Can you work these out from the model? Positions are in its coordinate system, mm. A direction names the side the tool comes from. Round coordinates to 2 decimals unless told otherwise and drop trailing zeros. Write each loop counter-clockwise with the first axis right and the second up, starting at its lowest first coordinate (ties: lowest second). Pieces come first, ordered by that corner, then holes. Notation, with made-up numbers: M 55.5,36.25 L 99.5,36.25 A20 cw 99.5,62.25 Z; hole C 48,45.5 d10. An arc over 180 degrees is marked long. Answer in a Markdown table with one row per item. Add a question column.
(1) Suppose I cut it at C-C, the plane z = -1.75. Write out the boundary of the cut face in (x, y).
(2) If I drill on probe 1 along X at (y, z) = (6.5, 8.5); probe 2 along X at (y, z) = (-1, -5.5); probe 3 along Z at (x, y) = (-15, 4.5), over which ranges is the centre line in solid material (lowest first)?
(3) Suppose I cut it at B-B, the plane y = 15. Write out the boundary of the cut face in (x, z), then the cut area to 3 significant figures.
(4) If we mould it in two halves opening along Y, with no side actions, what happens to faces 4 (the face through (0, -20, 0)), 5 (the face through (20.25, 0, 0)), 6 (the face through (-13, 10, -9))? For each: released by +Y, released by -Y, zero draft, split by the parting line, or undercut.
(5) For faces 1 (the face through (23.97, 12.54, -1.05)), 2 (the face through (-13, 0, 9)), 3 (the face through (-21.75, 7, 0)), which set-ups out of +Z, -Z, +X, -X, +Y, -Y let a thin tool reach every point of the face, with its end or its side?
(6) I'm going to push flat-ended pins straight in: pin 1 (0.6 mm diameter, centred on y = 4, z = -9, fed in from +X); pin 2 (4 mm diameter, centred on y = 6.5, z = 3, fed in from +X); pin 3 (10 mm diameter, centred on y = 1, z = -1, fed in from +X); pin 4 (1 mm diameter, centred on y = 3, z = 9, fed in from -X). Where does each tip first touch, or does it pass through?
(7) Suppose I cut it at A-A, the plane z = 8.75. Write out the boundary of the cut face in (x, y).
(8) Suppose I cut it at D-D, the plane y = 1. Write out the boundary of the cut face in (x, z).
from build123d import *

# Parameters (mm, degrees)
F0_W      = 40.5
F0_H      = 40
F1_DEPTH  = 10
F3_DEPTH  = 1.5
F4_R      = 2.75
F5_DEPTH  = 4.5
F7_DEPTH  = 1.5
F8_R      = 2.75
F9_DEPTH  = 4.5
F10_W     = 5
F10_H     = 10
F11_DEPTH = 2
F12_W     = 5
F12_H     = 10
F13_DEPTH = 2


with BuildPart() as f1:
    # F0 (on Top) → F1 (new body, symmetric)
    with BuildSketch(Plane.XY):
        Rectangle(F0_W, F0_H)
    extrude(amount=F1_DEPTH, both=True)

    # F2 (on face) → F3 (join)
    with BuildSketch(Plane(origin=(-20.25, 0, 0), x_dir=(0, -1, 0), z_dir=(-1, 0, 0))):
        with BuildLine():
            Line((-10, -6.5), (-10, 6.5))
            ThreePointArc((-10, 6.5), (-16.5, 0), (-10, -6.5))
        make_face()
        with BuildLine():
            ThreePointArc((-3.5, 0), (-5.4038059223, 4.5961940777), (-10, 6.5))
            Line((-10, 6.5), (-10, -6.5))
            ThreePointArc((-10, -6.5), (-5.4038059223, -4.5961940777), (-3.5, 0))
        make_face()
    extrude(amount=F3_DEPTH)

    # F4 (on face) → F5 (join)
    with BuildSketch(Plane(origin=(-21.75, 0, 0), x_dir=(0, -1, 0), z_dir=(-1, 0, 0))):
        with Locations((-10, 0)):
            Circle(F4_R)
    extrude(amount=F5_DEPTH)

    # F6 (on face) → F7 (join)
    with BuildSketch(Plane.YZ.offset(20.25)):
        with BuildLine():
            ThreePointArc((16.5, 0), (14.5961940777, 4.5961940777), (10, 6.5))
            Line((10, 6.5), (10, -6.5))
            ThreePointArc((10, -6.5), (14.5961940777, -4.5961940777), (16.5, 0))
        make_face()
        with BuildLine():
            Line((10, -6.5), (10, 6.5))
            ThreePointArc((10, 6.5), (3.5, 0), (10, -6.5))
        make_face()
    extrude(amount=F7_DEPTH)

    # F8 (on face) → F9 (join)
    with BuildSketch(Plane.YZ.offset(21.75)):
        with Locations((10, 0)):
            Circle(F8_R)
    extrude(amount=F9_DEPTH)

    # F10 (on face) → F11 (cut)
    with BuildSketch(Plane(origin=(0, 0, -10), x_dir=(1, 0, 0), z_dir=(0, 0, -1))):
        with Locations((-12.75, -5)):
            Rectangle(F10_W, F10_H)
    extrude(amount=-F11_DEPTH, mode=Mode.SUBTRACT)

    # F12 (on face) → F13 (cut)
    with BuildSketch(Plane.XY.offset(10)):
        with Locations((-12.75, 5)):
            Rectangle(F12_W, F12_H)
    extrude(amount=-F13_DEPTH, mode=Mode.SUBTRACT)


solid = f1.part
Calculated:
| question | item | result |
|---|---|---|
| 1 | outline | M -26.25,7.88 L -21.75,7.88 L -21.75,3.74 L -20.25,3.74 L -20.25,-20 L 20.25,-20 L 20.25,3.74 L 21.75,3.74 L 21.75,7.88 L 26.25,7.88 L 26.25,12.12 L 21.75,12.12 L 21.75,16.26 L 20.25,16.26 L 20.25,20 L -20.25,20 L -20.25,16.26 L -21.75,16.26 L -21.75,12.12 L -26.25,12.12 Z |
| 2 | probe 1 | -20.25 to -15.25, -10.25 to 20.25 |
| 2 | probe 2 | -20.25 to 20.25 |
| 2 | probe 3 | -8 to 8 |
| 3 | outline | M -21.75,-4.15 L -20.25,-4.15 L -20.25,-10 L 20.25,-10 L 20.25,-4.15 L 21.75,-4.15 L 21.75,4.15 L 20.25,4.15 L 20.25,10 L -20.25,10 L -20.25,4.15 L -21.75,4.15 Z |
| 3 | area | 835 mm² |
| 4 | face 4 | released by -Y |
| 4 | face 5 | zero draft |
| 4 | face 6 | undercut |
| 5 | face 1 | +X |
| 5 | face 2 | +Z |
| 5 | face 3 | -X |
| 6 | pin 1 | x = 20.25 |
| 6 | pin 2 | x = 26.25 |
| 6 | pin 3 | x = 21.75 |
| 6 | pin 4 | x = -20.25 |
| 7 | outline | M -20.25,-20 L 20.25,-20 L 20.25,20 L -20.25,20 Z; hole M -15.25,0 L -10.25,0 L -10.25,10 L -15.25,10 Z |
| 8 | outline | M -20.25,-10 L -15.25,-10 L -15.25,-8 L -10.25,-8 L -10.25,-10 L 20.25,-10 L 20.25,10 L -10.25,10 L -10.25,8 L -15.25,8 L -15.25,10 L -20.25,10 Z |
